Input: part model. Units: mm. Frame: model coordinates. Coordinates: 2 decimals unless noted, no trailing zeros. Order: outer loops, then holes, each group sorted by start corner. A loop starts at its lowest first (then second) coordinate and runs counter-clockwise, first axis right, second up. Notation, with made-up numbers: (1.25, 62) - (17.25, 62) arc R33 cw to (17.25, 95) - close; hole circle Ø4 at (13, 73). An arc over 180 degrees is marked (long way). Use a Markdown table: item, result. Add a question column.
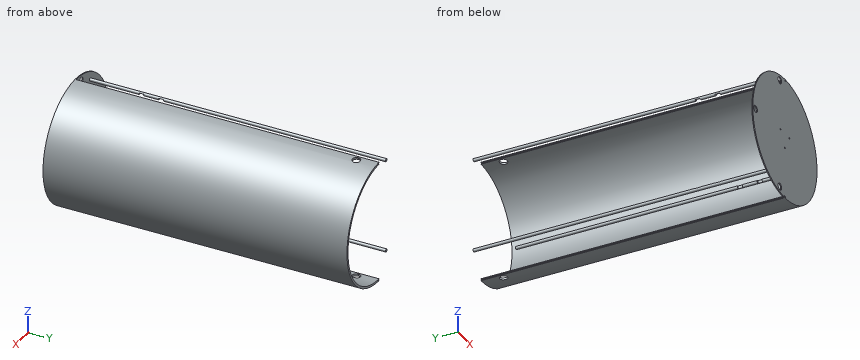
from build123d import *

# Parameters (mm, degrees)
SKETCH2_R               = 62.5
SKETCH2_R_2             = 0.75
BOSS_EXTRUDE1_DEPTH     = 1
SKETCH3_R               = 1.5
BOSS_EXTRUDE2_DEPTH     = 300
SKETCH5_W               = 3
SKETCH5_H               = 5
CUT_EXTRUDE1_DEPTH      = 5
CIRPATTERN1_COUNT       = 3
BOSS_EXTRUDE3_DEPTH     = 307
CUT_EXTRUDE2_REACH      = 322.432
SKETCH10_W              = 1.5
SKETCH10_H              = 1.5
SKETCH10_W_2            = 3
SKETCH11_R              = 3.5
CUT_EXTRUDE3_DEPTH      = 5
CIRPATTERN4_COUNT       = 2
CIRPATTERN4_ANGLE       = 80
MIRROR1_COPY_1_SKETCH_R = 3.5
MIRROR1_COPY_1_DEPTH    = 5
MIRROR1_COPY_2_SKETCH_R = 3.5
MIRROR1_COPY_2_DEPTH    = 5


with BuildPart() as part:
    # Sketch2 → Boss-Extrude1 (new body)
    with BuildSketch(Plane(origin=(0, 0, 0), x_dir=(1, 0, 0), z_dir=(0, 1, 0))):
        with Locations(Location((0, 0, 0), (0, 0, 270))):
            Circle(SKETCH2_R)
        with Locations(Location((0, 10, 0), (0, 0, 270))):
            Circle(SKETCH2_R_2, mode=Mode.SUBTRACT)
        with Locations(Location((8.660254038, -5, 0), (0, 0, 270))):
            Circle(SKETCH2_R_2, mode=Mode.SUBTRACT)
        with Locations(Location((-8.660254038, -5, 0), (0, 0, 270))):
            Circle(SKETCH2_R_2, mode=Mode.SUBTRACT)
    extrude(amount=BOSS_EXTRUDE1_DEPTH)

    # Sketch3 → Boss-Extrude2 (add)
    with BuildSketch(Plane(origin=(0, 1, 0), x_dir=(1, 0, 0), z_dir=(0, 1, 0))):
        with Locations(Location((55, 0, 0), (0, 0, 270))):
            Circle(SKETCH3_R)
    boss_extrude2 = extrude(amount=BOSS_EXTRUDE2_DEPTH)

    # Sketch5 → Cut-Extrude1 (cut)
    with BuildSketch(Plane(origin=(55, 0, 0), x_dir=(0, 0, -1), z_dir=(1, 0, 0))):
        with Locations((0, 53.5)):
            Rectangle(SKETCH5_W, SKETCH5_H)
        with Locations((0, 73.5)):
            Rectangle(SKETCH5_W, SKETCH5_H)
    cut_extrude1 = extrude(amount=-CUT_EXTRUDE1_DEPTH, mode=Mode.SUBTRACT)

    # CirPattern1: Boss-Extrude2, Cut-Extrude1 ×3 about axis
    cirpattern1_axis = Axis((0, 0, 0), (0, 1, 0))
    add([boss_extrude2.rotate(cirpattern1_axis, i * 360 / CIRPATTERN1_COUNT) for i in range(1, CIRPATTERN1_COUNT)])
    add([cut_extrude1.rotate(cirpattern1_axis, i * 360 / CIRPATTERN1_COUNT) for i in range(1, CIRPATTERN1_COUNT)], mode=Mode.SUBTRACT)

    # Sketch6 → Boss-Extrude3 (add)
    with BuildSketch(Plane(origin=(0, 1, 0), x_dir=(1, 0, 0), z_dir=(0, 1, 0))):
        with BuildLine():
            Line((0, 62.5), (0, 60.5))
            ThreePointArc((0, 60.5), (60.5, 0), (0, -60.5))
            Line((0, -60.5), (0, -62.5))
            ThreePointArc((0, -62.5), (62.5, 0), (0, 62.5))
        make_face()
    extrude(amount=BOSS_EXTRUDE3_DEPTH)

    # Sketch10 → Cut-Extrude2 (cut, up to next)
    with BuildSketch(Plane(origin=(0, 308, 0), x_dir=(1, 0, 0), z_dir=(0, 1, 0)), mode=Mode.PRIVATE) as cut_extrude2_sk1:
        with Locations((0.75, -61.5)):
            Rectangle(SKETCH10_W, SKETCH10_H)
    cut_extrude2_tool1 = extrude(cut_extrude2_sk1.sketch, amount=-CUT_EXTRUDE2_REACH, mode=Mode.PRIVATE) & part.part
    # Sketch10 → Cut-Extrude2 (cut, up to next)
    with BuildSketch(Plane(origin=(0, 308, 0), x_dir=(1, 0, 0), z_dir=(0, 1, 0)), mode=Mode.PRIVATE) as cut_extrude2_sk2:
        with Locations((0, 61.5)):
            Rectangle(SKETCH10_W_2, SKETCH10_H)
    cut_extrude2_tool2 = extrude(cut_extrude2_sk2.sketch, amount=-CUT_EXTRUDE2_REACH, mode=Mode.PRIVATE) & part.part
    add(cut_extrude2_tool1.solids().sort_by_distance((0.75, 308, 61.5))[0], mode=Mode.SUBTRACT)
    add(cut_extrude2_tool2.solids().sort_by_distance((0, 308, -61.5))[0], mode=Mode.SUBTRACT)

    # Sketch11 → Cut-Extrude3 (cut)
    with BuildSketch(Plane(origin=(0, 1, 0), x_dir=(1, 0, 0), z_dir=(0, 1, 0))):
        with Locations(Location((-57, 0, 0), (0, 0, 270))):
            Circle(SKETCH11_R)
    cut_extrude3 = extrude(amount=-CUT_EXTRUDE3_DEPTH, mode=Mode.SUBTRACT)

    # CirPattern4: Cut-Extrude3 ×2 about axis
    cirpattern4_axis = Axis((0, 1, 0), (0, 1, 0))
    for i in range(1, CIRPATTERN4_COUNT):
        add(cut_extrude3.rotate(cirpattern4_axis, i * CIRPATTERN4_ANGLE / (CIRPATTERN4_COUNT - 1)), mode=Mode.SUBTRACT)

    # Mirror1 copy 1 sketch → Mirror1 copy 1 (cut)
    with BuildSketch(Plane(origin=(0, 1, 0), x_dir=(0.17364817766692714, 0, 0.9848077530122086), z_dir=(0, 1, 0))):
        with Locations((-57, 0)):
            Circle(MIRROR1_COPY_1_SKETCH_R)
    extrude(amount=-MIRROR1_COPY_1_DEPTH, mode=Mode.SUBTRACT)

    # Mirror1 copy 2 sketch → Mirror1 copy 2 (cut)
    with BuildSketch(Plane(origin=(0, 1, 0), x_dir=(1, 0, 0), z_dir=(0, 1, 0))):
        with Locations((-57, 0)):
            Circle(MIRROR1_COPY_2_SKETCH_R)
    extrude(amount=-MIRROR1_COPY_2_DEPTH, mode=Mode.SUBTRACT)

    # Sketch16 → CBORE for #6 Binding Head Machine Screw1 (revolve, cut)
    with BuildSketch(Plane(origin=(5.561206614, 287.931721959, 62.252092182), x_dir=(0.9960334749074581, 0, -0.08897930581755542), z_dir=(0, 1, 0))):
        Polygon((0, 0), (0, 8.293442612), (2.15265, 7), (2.15265, 2.2098), (3.96875, 2.2098), (3.96875, 0), align=None)
    cbore_for_6_binding_head_machine_screw1 = revolve(axis=Axis((6.126225206, 287.931721959, 68.576904747), (-0.08897930581755542, 0, -0.9960334749074581)), mode=Mode.SUBTRACT)

    # Mirror3: CBORE for #6 Binding Head Machine Screw1 across plane
    add(cbore_for_6_binding_head_machine_screw1.mirror(Plane.XY), mode=Mode.SUBTRACT)


solid = part.part
1) Cut plane C-C (z = -24). Return the cut outline in (x, y), and give its area (3 significant figures).
2) Material intervals for L1, parallel to Y at x = -3, z = 18; L2, parallel to X at y = 0.3, z = -10; L3, parallel to X at y = 0.2, z = 0, sorted ascending.
3) Cut plane D-D (x = 32). Return the cut outline in (y, z), and give its area (3 significant figures).
4) Contact query for flat-ended pins moving along their axis: P1, Ø1.8, axis at x = -28, z = 48, coming from the +Y side; P2, Ø1, axis at y = 202.5, z = -18.5, coming from the -X side; P3, Ø11, axis at x = -9.9, z = -56.13, coming from the +Y side. Output: stop coordinate, or through.
5) Cut plane B-B (x = -57). Return the cut outline in (y, z), and give its area (3 significant figures).
6) Cut plane A-A (y = 103.5). Return the cut outline in (x, z), and give its area (3 significant figures).
Computed:
| question | item | result |
|---|---|---|
| 1 | outline | (-57.71, 0) - (57.71, 0) - (57.71, 308) - (55.54, 308) - (55.54, 1) - (-57.71, 1) - close |
| 1 | area | 782 mm2 |
| 2 | L1 | y = 0 to 1 |
| 2 | L2 | x = -61.69 to -0.75, 0.75 to 61.69 |
| 2 | L3 | x = -62.5 to -60.5, -53.5 to 62.5 |
| 3 | outline | (0, -53.69) - (308, -53.69) - (308, -51.34) - (1, -51.34) - (1, 51.34) - (308, 51.34) - (308, 53.69) - (0, 53.69) - close |
| 3 | area | 1,550 mm2 |
| 4 | P1 | stops at y = 301 |
| 4 | P2 | stops at x = 57.44 |
| 4 | P3 | stops at y = 1 |
| 5 | outline | (0, -25.64) - (1, -25.64) - (1, -3.5) - (0, -3.5) - close; (0, 3.5) - (1, 3.5) - (1, 25.64) - (0, 25.64) - close |
| 5 | area | 44.3 mm2 |
| 6 | outline | circle Ø3 at (-27.5, -47.63); circle Ø3 at (-27.5, 47.63); (0, -62.5) arc R62.5 ccw to (0, 62.5) - (0, 62.25) - (1.5, 62.25) - (1.5, 60.75) - (0, 60.75) - (0, 60.5) arc R60.5 cw to (0, -60.5) - (0, -60.75) - (1.5, -60.75) - (1.5, -62.25) - (0, -62.25) - close; circle Ø3 at (55, 0) |
| 6 | area | 403 mm2 |
